Input: part model. Units: mm. Frame: model coordinates. Coordinates: 2 decimals unless noted, no trailing zeros. Write each loop counter-clockwise with the first axis right and the second up, starting at its lowest first coordinate (ties: lowest second). Pieces come first, ordered by that corner, then holes. Notation, with made-up numbers: M 67,-17 L 97,-17 A32 cw 97,16 Z; hole C 89,22.25 d11. An arc over 180 degrees is marked long. Use one line per item in the form item = value.
from build123d import *

# Parameters (mm, degrees)
BOSS_EXTRUDE1_DEPTH = 3.175
SKETCH2_R           = 12.7
CUT_EXTRUDE1_DEPTH  = 76.2
FILLET1_R           = 30.48


with BuildPart() as part:
    # Sketch1 → Boss-Extrude1 (new body)
    with BuildSketch(Plane(origin=(0, 0, 0), x_dir=(1, 0, 0), z_dir=(0, 1, 0))):
        with BuildLine():
            Line((211.534409722, 68.311873697), (-33.027609136, 198.909430038))
            ThreePointArc((-33.027609136, 198.909430038), (-68.829570139, 198.316531428), (-87.244015898, 167.607572999))
            Line((-87.244015898, 167.607572999), (-96.424223864, -109.488126303))
            Line((-96.424223864, -109.488126303), (211.534409722, 68.311873697))
        make_face()
    extrude(amount=BOSS_EXTRUDE1_DEPTH)

    # Sketch2 → Cut-Extrude1 (cut)
    with BuildSketch(Plane(origin=(0, 3.175, 0), x_dir=(1, 0, 0), z_dir=(0, 1, 0))):
        with Locations(Location((-42.355812517, 152.46263816, 0), (0, 0, 270))):
            Circle(SKETCH2_R)
    extrude(amount=-CUT_EXTRUDE1_DEPTH, mode=Mode.SUBTRACT)

    # Fillet1
    fillet1_edges = [part.edges().sort_by_distance(p)[0] for p in [
        (211.534409722, 1.5875, -68.311873697),
        (-96.424223864, 1.5875, 109.488126303),
    ]]
    fillet(fillet1_edges, radius=FILLET1_R)


solid = part.part
(1) Section query B-B on x = 23.5. Return the cut outline in (y, z) (3 decimals), plus the area to 3 significant figures.
Computed:
outline = M 0,-168.723 L 3.175,-168.723 L 3.175,40.25 L 0,40.25 Z
area = 663 mm^2
(2) Section query A-A on y = 2.6. Return the cut outline in (x, z).
Computed:
outline = M -94.61,54.65 L -87.24,-167.61 A36.87 ccw -33.03,-198.91 L 163.13,-94.16 A30.48 ccw 164.01,-40.88 L -48.9,82.05 A30.48 ccw Z; hole C -42.36,-152.46 d25.4
(3) Line query: probe 1 along Z at (x, y) = (-44, 2.5); probe 2 along X at (y, z) = (2.7, -155); probe 3 along Z at (x, y) = (-32.5, 2.35). Output: solid intervals per line, ascending.
Computed:
probe_1 = -202.7 to -165.06, -139.87 to 79.22
probe_2 = -87.66 to -54.8, -29.91 to 49.2
probe_3 = -198.63 to -160.47, -144.45 to 72.58
(4) Section query C-C on z = 3. Return the cut outline in (x, y) (3 decimals), plus the area to 3 significant figures.
Computed:
outline = M -92.896,0 L 88.019,0 L 88.019,3.175 L -92.896,3.175 Z
area = 574 mm^2
(5) First-contact query: pin 1 Ø1 at (x, y) = (151, 1.5) entering from -Z; pin 2 Ø1 at (y, z) = (2, 40.5) entering from -X; pin 3 Ø23 at (x, z) = (-42.36, -152.46) entering from +Y (1 decimal). Flat tips, straight axial feed; report the tip coordinate or a pass-through.
Computed:
pin_1 = -100.9
pin_2 = -94.16
pin_3 = through
